from build123d import *

# Parameters (mm, degrees)
BOSS_EXTRUDE1_DEPTH = 122
SKETCH2_R           = 2.75
CUT_EXTRUDE1_DEPTH  = 20.65
SKETCH3_R           = 2.55
CUT_EXTRUDE2_DEPTH  = 20.95


with BuildPart() as part:
    # Sketch1 → Boss-Extrude1 (new body)
    with BuildSketch(Plane.XY):
        Polygon((0, 18.15), (0, 0), (18.45, 0), (18.45, -1.5), (-1.5, -1.5), (-1.5, 18.15), align=None)
    extrude(amount=BOSS_EXTRUDE1_DEPTH)

    # Sketch2 → Cut-Extrude1 (cut, through all)
    with BuildSketch(Plane(origin=(0, -1.5, 0), x_dir=(-1, 0, 0), z_dir=(0, -1, 0))):
        with Locations((-13.95, -107)):
            Circle(SKETCH2_R)
        with Locations((-13.95, -78.76)):
            Circle(SKETCH2_R)
    extrude(amount=-CUT_EXTRUDE1_DEPTH, mode=Mode.SUBTRACT)

    # Sketch3 → Cut-Extrude2 (cut, through all)
    with BuildSketch(Plane.ZY.offset(1.5)):
        with Locations((30, 12.15)):
            Circle(SKETCH3_R)
        with Locations((70.64, 12.15)):
            Circle(SKETCH3_R)
    extrude(amount=-CUT_EXTRUDE2_DEPTH, mode=Mode.SUBTRACT)


solid = part.part
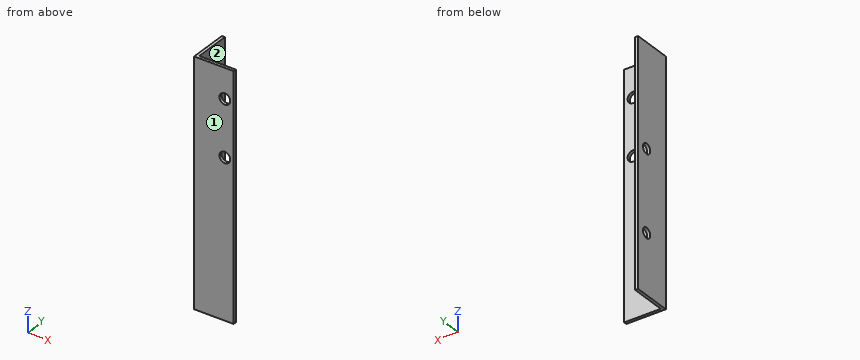
For this review, take the finished solid that the model builds, in its own axes (mm). Face numbers are marked on the shaded views. A direction names the side the tool comes from. Round coordinates to 2 decimals unless told otherwise and drop trailing zeros. Loops run counter-clockwise (first coordinate to the right, second up) from the corner with the lowest first, then second, coordinate; pieces in that order, holes last. Notation, with made-up numbers: (45.25, 8) - (70.25, 8) arc R34 cw to (70.25, 39) - close; hole circle Ø8 at (27.25, -27). An arc over 180 degrees is marked (long way). One line per item, written item: value. Start each with the question number.
Item 1: For L1, parallel to Z at x = 13.95, y = -1.15; L2, parallel to Y at x = -0.5, z = 70.64; L3, parallel to X at y = -1.05, z = 107, list the stretches that pass through material, from the lowest coordinate up.
Item 2: Take a section at A-A (z = 78.76). Give the boundary of the cut face in (x, y), plus the area to 3 significant figures.
Item 3: Take a section at C-C (y = 12.15). Give the boundary of the cut face in (x, z), plus the area to 3 significant figures.
Item 4: Clearance check with flat-ended pins moving along their axes: pin 1 Ø2 at (x, z) = (14.5, 92) entering from +Y; pin 2 Ø6.5 at (x, z) = (13.95, 78.76) entering from -Y; pin 3 Ø5 at (y, z) = (15.5, 91) entering from +X. State where each tip first meets the part, or that it passes through.
Item 5: Take a section at D-D (z = 30). Give the boundary of the cut face in (x, y).
Item 6: Take a section at B-B (x = 13.95). Give the boundary of the cut face in (y, z).
Item 7: For the marked faces 1 and 2, list the 3-axis set-ups (+Z, -Z, +X, -X, +Y, -Y) from which the entire face can be reached by the end or side of a thin tool; tool diameter is ignored.
Answer below:
1. L1: z = 0 to 76.01, 81.51 to 104.25, 109.75 to 122
1. L2: y = -1.5 to 9.6, 14.7 to 18.15
1. L3: x = -1.5 to 11.2, 16.7 to 18.45
2. outline: (-1.5, -1.5) - (11.2, -1.5) - (11.2, 0) - (0, 0) - (0, 18.15) - (-1.5, 18.15) - close; (16.7, -1.5) - (18.45, -1.5) - (18.45, 0) - (16.7, 0) - close
2. area: 48.9 mm2
3. outline: (-1.5, 0) - (0, 0) - (0, 27.45) - (-1.5, 27.45) - close; (-1.5, 32.55) - (0, 32.55) - (0, 68.09) - (-1.5, 68.09) - close; (-1.5, 73.19) - (0, 73.19) - (0, 122) - (-1.5, 122) - close
3. area: 168 mm2
4. pin 1: stops at y = 0
4. pin 2: stops at y = -1.5
4. pin 3: stops at x = 0
5. outline: (-1.5, -1.5) - (18.45, -1.5) - (18.45, 0) - (0, 0) - (0, 9.6) - (-1.5, 9.6) - close; (-1.5, 14.7) - (0, 14.7) - (0, 18.15) - (-1.5, 18.15) - close
6. outline: (-1.5, 0) - (0, 0) - (0, 76.01) - (-1.5, 76.01) - close; (-1.5, 81.51) - (0, 81.51) - (0, 104.25) - (-1.5, 104.25) - close; (-1.5, 109.75) - (0, 109.75) - (0, 122) - (-1.5, 122) - close
7. face 1: +Z, -Z, +X, -X, -Y
7. face 2: +Z, -Z, +X, +Y
